Could you check a few things on this model? Use its own coordinates, in mm. Give positions to 0.01 mm unless a question says otherwise; leave off trailing zeros. Loops run counter-clockwise (first coordinate to the right, second up) from the corner with the lowest first, then second, coordinate; pieces in that order, holes last. Notation, with made-up numbers: (48, -10.75) - (85, -10.75) arc R29 cw to (85, 23.25) - close; hole circle Ø8 at (-3.5, 35). An arc over 180 degrees is marked (long way). Use CSV: the item, a comma, the result in double quotes.
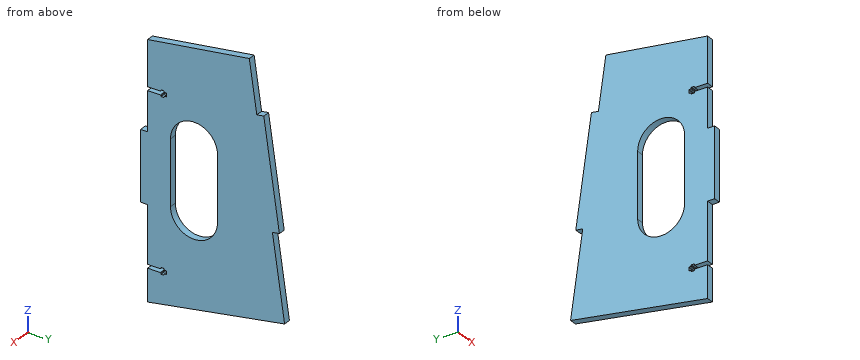
from build123d import *

# Parameters (mm, degrees)
BOSS_EXTRUDE1_DEPTH = 6
CUT_EXTRUDE1_DEPTH  = 6
CUT_EXTRUDE2_DEPTH  = 6
SKETCH5_W           = 3.1
SKETCH5_H           = 16
CUT_EXTRUDE3_DEPTH  = 257.585419281
SKETCH6_W           = 5.5
SKETCH6_H           = 2.8
CUT_EXTRUDE4_DEPTH  = 257.585419281
FILLET1_R           = 0.4
CUT_EXTRUDE5_DEPTH  = 257.585419281


with BuildPart() as part:
    # Sketch1 → Boss-Extrude1 (new body)
    with BuildSketch(Plane(origin=(0, 0, 0), x_dir=(0, 0, -1), z_dir=(1, 0, 0))):
        Polygon((-8.423886954, 100.420733136), (5.846423254, 2.80742232), (224.813620111, 2.80742232), (203.793040966, 125.38142721), (199.85477244, 130.869460409), align=None)
    extrude(amount=BOSS_EXTRUDE1_DEPTH)

    # Sketch2 → Cut-Extrude1 (cut)
    with BuildSketch(Plane(origin=(6, 0, 0), x_dir=(0, 0, -1), z_dir=(1, 0, 0))):
        Polygon((5.846423254, 2.80742232), (85.846423254, 2.80742232), (85.846423254, 8.80742232), (4.969269713, 8.80742232), align=None)
        Polygon((144.813620111, 2.80742232), (144.813620111, 8.80742232), (223.78466234, 8.80742232), (224.813620111, 2.80742232), align=None)
        Polygon((41.050223347, 107.653464977), (41.918151168, 101.716571741), (-7.555959133, 94.4838399), (-8.423886954, 100.420733136), align=None)
        Polygon((131.999265462, 120.949510704), (132.867193283, 115.012617467), (203.793040966, 125.38142721), (199.85477244, 130.869460409), align=None)
    extrude(amount=-CUT_EXTRUDE1_DEPTH, mode=Mode.SUBTRACT)

    # Sketch4 → Cut-Extrude2 (cut)
    with BuildSketch(Plane(origin=(6, 0, 0), x_dir=(0, 0, -1), z_dir=(1, 0, 0))):
        Polygon((-7.555959133, 94.4838399), (-1.619065897, 95.351767721), (11.033047276, 8.80742232), (4.969269713, 8.80742232), align=None)
    extrude(amount=-CUT_EXTRUDE2_DEPTH, mode=Mode.SUBTRACT)

    # Sketch5 → Cut-Extrude3 (cut, through all)
    with BuildSketch(Plane(origin=(6, 0, 0), x_dir=(0, 0, -1), z_dir=(1, 0, 0))):
        with Locations((50.846423254, 16.80742232)):
            Rectangle(SKETCH5_W, SKETCH5_H)
        with Locations((194.813620111, 16.80742232)):
            Rectangle(SKETCH5_W, SKETCH5_H)
    extrude(amount=-CUT_EXTRUDE3_DEPTH, mode=Mode.SUBTRACT)

    # Sketch6 → Cut-Extrude4 (cut, through all)
    with BuildSketch(Plane(origin=(6, 0, 0), x_dir=(0, 0, -1), z_dir=(1, 0, 0))):
        with Locations((50.846423254, 21.40742232)):
            Rectangle(SKETCH6_W, SKETCH6_H)
        with Locations((194.813620111, 21.40742232)):
            Rectangle(SKETCH6_W, SKETCH6_H)
    extrude(amount=-CUT_EXTRUDE4_DEPTH, mode=Mode.SUBTRACT)

    # Fillet1
    fillet1_edges = [part.edges().sort_by_distance(p)[0] for p in [
        (3, 24.80742232, -193.263620111),
        (3, 24.80742232, -196.363620111),
        (3, 20.00742232, -52.396423254),
        (3, 22.80742232, -52.396423254),
        (3, 20.00742232, -196.363620111),
        (3, 22.80742232, -196.363620111),
        (3, 22.80742232, -49.296423254),
        (3, 22.80742232, -48.096423254),
        (3, 20.00742232, -49.296423254),
        (3, 20.00742232, -53.596423254),
        (3, 20.00742232, -48.096423254),
        (3, 22.80742232, -53.596423254),
        (3, 22.80742232, -193.263620111),
        (3, 22.80742232, -192.063620111),
        (3, 20.00742232, -193.263620111),
        (3, 20.00742232, -197.563620111),
        (3, 20.00742232, -192.063620111),
        (3, 22.80742232, -197.563620111),
        (3, 24.80742232, -49.296423254),
        (3, 24.80742232, -52.396423254),
    ]]
    fillet(fillet1_edges, radius=FILLET1_R)

    # Sketch7 → Cut-Extrude5 (cut, through all)
    with BuildSketch(Plane(origin=(6, 0, 0), x_dir=(0, 0, -1), z_dir=(1, 0, 0))):
        with BuildLine():
            Line((85.173180011, 68.290188576), (140.173180011, 68.290188576))
            ThreePointArc((140.173180011, 68.290188576), (160.173180011, 48.290188576), (140.173180011, 28.290188576))
            Line((140.173180011, 28.290188576), (85.173180011, 28.290188576))
            ThreePointArc((85.173180011, 28.290188576), (65.173180011, 48.290188576), (85.173180011, 68.290188576))
        make_face()
    extrude(amount=-CUT_EXTRUDE5_DEPTH, mode=Mode.SUBTRACT)


solid = part.part
1) Suppose I cut it at D-D (y = 75). Please give me the cut outline in (x, z).
Answer below:
outline,"(0, -212.43) - (6, -212.43) - (6, -1.36) - (0, -1.36) - close"
2) I need wall thicknesses on line 1 along Z through (x, y) = (5.55, 30); line 2 along Y through (x, z) = (0.9, -122); line 3 along Y through (x, z) = (0.9, -139). Which ranges of each line are inside material? Lowest first, please.
Answer below:
line 1,"z = -220.15 to -148.26, -77.08 to -7.93"
line 2,"y = 2.81 to 28.29, 68.29 to 119.49"
line 3,"y = 2.81 to 28.29, 68.29 to 115.91"
3) Suppose I cut it at B-B (y = 40). Please give me the cut outline in (x, z), plus the area to 3 significant figures.
Answer below:
outline,"(0, -218.44) - (6, -218.44) - (6, -158.37) - (0, -158.37) - close; (0, -66.97) - (6, -66.97) - (6, -6.47) - (0, -6.47) - close"
area,"723 mm2"
4) I'm going to push flat-ended pins straight in: P1, Ø1.8, axis at x = 1.5, y = 14.5, coming from the +Z side; P2, Ø1.6, axis at x = 2, y = 22, coming from the +Z side; P3, Ø2, axis at x = 4, z = -177.5, coming from the -Y side. Where does each tip first touch, or does it pass through?
Answer below:
P1,"stops at z = -10.07"
P2,"stops at z = -8.99"
P3,"stops at y = 8.81"
5) Suppose I cut it at A-A (z = -118). Please give me the cut outline in (x, y), plus the area to 3 significant figures.
Answer below:
outline,"(0, 2.81) - (6, 2.81) - (6, 28.29) - (0, 28.29) - close; (0, 68.29) - (6, 68.29) - (6, 118.9) - (0, 118.9) - close"
area,"457 mm2"
6) Suppose I cut it at C-C (z = -168). Please give me the cut outline in (x, y), plus the area to 3 significant figures.
Answer below:
outline,"(0, 8.81) - (6, 8.81) - (6, 120.15) - (0, 120.15) - close"
area,"668 mm2"
